Source: CAD feature listing. Evaluate the final solid. Frame: model axes, mm. Face numbers are marked on the shaded views. A direction names the side the tool comes from. Round coordinates to 2 decimals unless told otherwise and drop trailing zeros. Write each loop counter-clockwise with the first axis right and the second up, starting at its lowest first coordinate (ties: lowest second). Pieces come first, ordered by that corner, then holes. Notation, with made-up numbers: M 1,31.25 L 22,31.25 A21 ccw 22,51.25 Z; hole C 48.5,5 d1. An arc over 180 degrees is marked long. Answer in a Markdown table with one row per item. Add a question column.
Item 1: Cut plane A-A on y = 20. Return loops of the section in (x, z).
Item 2: Cut plane C-C on x = 121. Return loops of the section in (y, z), and give its area (3 significant figures).
Item 3: Cut plane D-D on z = 23.5. Return loops of the section in (x, y), and give its area (3 significant figures).
Item 4: Material intervals for probe 1 along Z at (x, y) = (-47, 22.5); probe 2 along Z at (x, y) = (-55, 20.25); probe 3 along X at (y, z) = (20.5, 124.5), sorted ascending.
Item 5: Contact query for flat-ended pins moving along their axis: pin 1 (12 mm diameter, centred on x = -45, y = 32, fed in from -Z); pin 2 (14 mm diameter, centred on x = 117, z = 42, fed in from +Y); pin 3 (3 mm diameter, centred on x = 12.5, y = 28, fed in from +Z). Output: stop coordinate, or through.
Item 6: Set-up query: the marked faces 1 and 2. Return all of +Z, -Z, +X, -X, +Y, -Y with unobstructed straight access to the full face (end or side cutting, diameter ignored); none if empty.
Item 7: Mould query, pull axis X, two halves, no side actions, for the marked faces 3, 4 and 5. Classes: released by +X, released by -X, zero draft, split by the parting line, or undercut.
Item 8: Cut plane B-B on x = -67. Return loops of the section in (y, z), and give its area (3 significant figures).
from build123d import *

# Parameters (mm, degrees)
SKETCH2_W           = 300
SKETCH2_H           = 300
BOSS_EXTRUDE1_DEPTH = 10
BOSS_EXTRUDE3_DEPTH = 30
SKETCH2_2_W         = 300
SKETCH2_2_H         = 300
CUT_EXTRUDE1_DEPTH  = 10
BOSS_EXTRUDE4_DEPTH = 5


with BuildPart() as part:
    # Sketch2 → Boss-Extrude1 (new body)
    with BuildSketch(Plane(origin=(0, 0, 0), x_dir=(1, 0, 0), z_dir=(0, 1, 0))):
        with Locations((20.355411955, -44.224555735)):
            Rectangle(SKETCH2_W, SKETCH2_H)
    extrude(amount=BOSS_EXTRUDE1_DEPTH)

    # Sketch7 → Boss-Extrude3 (add)
    # profile 1 of 4: a face of its own
    with BuildSketch(Plane(origin=(0, 10, 0), x_dir=(1, 0, 0), z_dir=(0, 1, 0))):
        Polygon((81.307092119, -68.428552611), (80.429718136, -29.428552611), (140.429718136, -28.078746484), (141.307092119, -67.078746484), align=None)
        Polygon((88.664625709, -62.011450502), (133.653242675, -60.999351988), (133.045983567, -34.006181808), (88.0573666, -35.018280322), align=None, mode=Mode.SUBTRACT)
    # profile 2 of 4: a face of its own
    with BuildSketch(Plane(origin=(0, 10, 0), x_dir=(1, 0, 0), z_dir=(0, 1, 0))):
        Polygon((-46.470752527, -180.781592729), (-80.941936453, -162.540499595), (-52.878716247, -109.507908939), (-18.407532321, -127.749002073), align=None)
        Polygon((-51.304328835, -118.826374708), (-72.351743989, -158.6008177), (-48.487078194, -171.229266792), (-27.43966304, -131.454823801), align=None, mode=Mode.SUBTRACT)
    # profile 3 of 4: a face of its own
    with BuildSketch(Plane(origin=(0, 10, 0), x_dir=(1, 0, 0), z_dir=(0, 1, 0))):
        Polygon((-53.708567917, 6.717259125), (-86.123521283, 57.207563128), (-53.304823682, 78.277282816), (-20.889870316, 27.786978813), align=None)
        Polygon((-29.78039362, 30.991833782), (-54.091608645, 68.859561784), (-76.812245446, 54.27283277), (-52.501030421, 16.405104768), align=None, mode=Mode.SUBTRACT)
    # profile 4 of 4: a face of its own
    with BuildSketch(Plane(origin=(0, 10, 0), x_dir=(1, 0, 0), z_dir=(0, 1, 0))):
        Polygon((81.307092119, -68.428552611), (12.159859746, -69.984141911), (-18.407532321, -127.749002073), (-52.878716247, -109.507908939), (-19.539590898, -46.505153929), (-53.708567917, 6.717259125), (-20.889870316, 27.786978813), (16.762252316, -30.86086487), (80.429718136, -29.428552611), align=None)
    extrude(amount=BOSS_EXTRUDE3_DEPTH)

    # Sketch2_2 → Cut-Extrude1 (cut)
    with BuildSketch(Plane(origin=(0, 0, 0), x_dir=(1, 0, 0), z_dir=(0, 1, 0))):
        with Locations((20.355411955, -44.224555735)):
            Rectangle(SKETCH2_2_W, SKETCH2_2_H)
    extrude(amount=CUT_EXTRUDE1_DEPTH, mode=Mode.SUBTRACT)

    # Sketch7_3 → Boss-Extrude4 (add)
    with BuildSketch(Plane(origin=(0, 10, 0), x_dir=(1, 0, 0), z_dir=(0, 1, 0))):
        Polygon((-27.43966304, -131.454823801), (-51.304328835, -118.826374708), (-72.351743989, -158.6008177), (-48.487078194, -171.229266792), align=None)
        Polygon((-52.501030421, 16.405104768), (-29.78039362, 30.991833782), (-54.091608645, 68.859561784), (-76.812245446, 54.27283277), align=None)
        Polygon((88.0573666, -35.018280322), (88.664625709, -62.011450502), (133.653242675, -60.999351988), (133.045983567, -34.006181808), align=None)
    extrude(amount=BOSS_EXTRUDE4_DEPTH)


solid = part.part
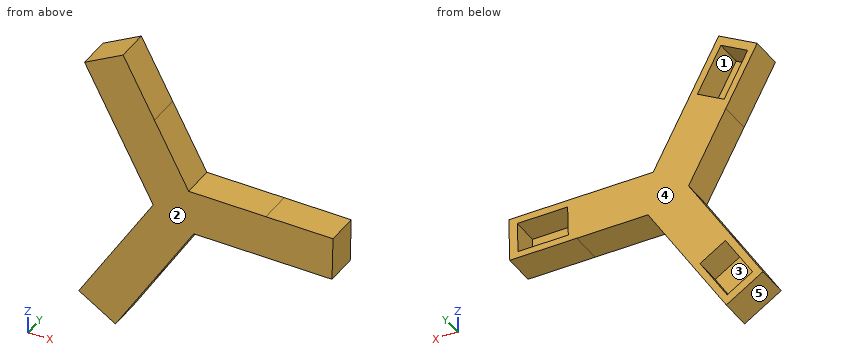
Results below:
| question | item | result |
|---|---|---|
| 1 | outline | M -86.12,-57.21 L -53.3,-78.28 L 16.76,30.86 L 140.43,28.08 L 141.31,67.08 L 12.16,69.98 L -46.47,180.78 L -80.94,162.54 L -19.54,46.51 Z; hole M -76.81,-54.27 L -54.09,-68.86 L -29.78,-30.99 L -52.5,-16.41 Z; hole M -72.35,158.6 L -51.3,118.83 L -27.44,131.45 L -48.49,171.23 Z; hole M 88.06,35.02 L 133.05,34.01 L 133.65,61 L 88.66,62.01 Z |
| 2 | outline | M 10,28.52 L 40,28.52 L 40,34.28 L 15,34.28 L 15,61.28 L 40,61.28 L 40,67.54 L 10,67.54 Z |
| 2 | area | 495 mm2 |
| 3 | outline | M -34.31,10 L 12.04,10 L 12.04,40 L -34.31,40 Z |
| 3 | area | 1,390 mm2 |
| 4 | probe 1 | -68.46 to -57.81, -19.94 to 3.73, 98.4 to 121.1, 168.42 to 180.5 |
| 4 | probe 2 | -77.19 to -68.28, -20.3 to -8.73, 113.52 to 125.81, 167.78 to 176.27 |
| 4 | probe 3 | -60.81 to -54.31, -40.58 to -16.69 |
| 5 | pin 1 | z = -74.69 |
| 5 | pin 2 | y = 15 |
| 5 | pin 3 | z = 72.18 |
| 6 | face 1 | +Y |
| 6 | face 2 | +Z, -Z, +X, -X, -Y |
| 7 | face 3 | undercut |
| 7 | face 4 | zero draft |
| 7 | face 5 | released by -X |
| 8 | outline | M 10,-69.48 L 40,-69.48 L 40,-60.57 L 15,-60.57 L 15,-38.99 L 40,-38.99 L 40,-27.42 L 10,-27.42 Z; M 10,136.19 L 40,136.19 L 40,148.49 L 15,148.49 L 15,161.43 L 40,161.43 L 40,169.92 L 10,169.92 Z |
| 8 | area | 1,410 mm2 |
